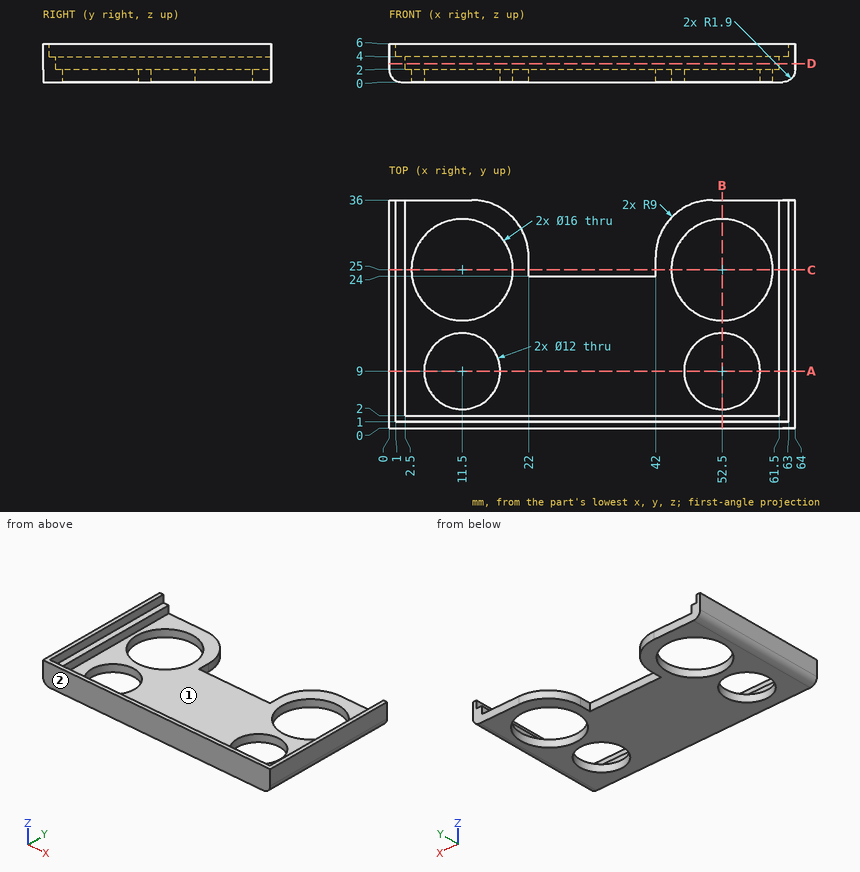
Source: three-view drawing plus pictorial views. Frame: mm from the lowest corner of the part. Round coordinates to 2 decimals unless told otherwise and drop trailing zeros. Order: outer loops, then holes, each group sorted by start corner. A loop starts at its lowest first (then second) coordinate and runs counter-clockwise, first axis right, second up. Notation, with made-up numbers: (-13, 88) - (40, 88) arc R24 cw to (40, 119) - close; hole circle Ø5 at (0, 85.5). An arc over 180 degrees is marked (long way). Use a Markdown table: item, result.
1. Mould query, pull axis X, two halves, no side actions, for the marked faces 1 and 2. Classes: +X half, -X half, draft (parallel to the pull), parting line (faces both ways), or undercut.
Evaluation:
| item | result |
|---|---|
| face 1 | undercut |
| face 2 | draft |
2. First-contact query: pin 1 (1.6 mm diameter, centred on y = 25.5, z = 1, fed in from +X); pin 2 (1.5 mm diameter, centred on x = 27, z = 2, fed in from -Y); pin 3 (18.5 mm diameter, centred on x = 11.5, y = 25, fed in from +Z); pin 4 (17 mm diameter, centred on x = 37, y = 19.5, fed in from +Z). Flat tips, straight axial feed; report the tip coordinate or a pass-through.
Evaluation:
| item | result |
|---|---|
| pin 1 | x = 64 |
| pin 2 | y = 0 |
| pin 3 | z = 4 |
| pin 4 | z = 2 |
3. Section C-C on y = 25. Return the cut outline in (x, z), then the cut area to 3 significant figures.
Evaluation:
| item | result |
|---|---|
| outline | (0, 1.9) arc R1.9 ccw to (1.9, 0) - (3.5, 0) - (3.5, 2) - (2.5, 2) - (2.5, 4) - (1, 4) - (1, 6) - (0, 6) - close; (19.5, 0) - (22, 0) - (22, 2) - (19.5, 2) - close; (42, 0) - (44.5, 0) - (44.5, 2) - (42, 2) - close; (60.5, 0) - (62.1, 0) arc R1.9 ccw to (64, 1.9) - (64, 6) - (63, 6) - (63, 4) - (61.5, 4) - (61.5, 2) - (60.5, 2) - close |
| area | 36.5 mm^2 |
4. Section B-B on x = 52.5. Return the cut outline in (y, z), then the cut area to 3 significant figures.
Evaluation:
| item | result |
|---|---|
| outline | (0, 0) - (3, 0) - (3, 2) - (2, 2) - (2, 4) - (1, 4) - (1, 6) - (0, 6) - close; (15, 0) - (17, 0) - (17, 2) - (15, 2) - close; (33, 0) - (36, 0) - (36, 2) - (33, 2) - close |
| area | 22.0 mm^2 |
5. Material intervals for probe 1 along Y at (x, z) = (52.5, 0.95); probe 2 along X at (y, z) = (6, 1.8); probe 3 along X at (y, z) = (27, 2.8), sorted ascending.
Evaluation:
| item | result |
|---|---|
| probe 1 | 0 to 3, 15 to 17, 33 to 36 |
| probe 2 | 0 to 6.3, 16.7 to 47.3, 57.7 to 64 |
| probe 3 | 0 to 2.5, 61.5 to 64 |
6. Section D-D on z = 2.9. Return the cut outline in (x, y).
Evaluation:
| item | result |
|---|---|
| outline | (0, 0) - (64, 0) - (64, 36) - (61.5, 36) - (61.5, 2) - (2.5, 2) - (2.5, 36) - (0, 36) - close |
7. Section A-A on y = 9. Return the cut outline in (x, z).
Evaluation:
| item | result |
|---|---|
| outline | (0, 1.9) arc R1.9 ccw to (1.9, 0) - (5.5, 0) - (5.5, 2) - (2.5, 2) - (2.5, 4) - (1, 4) - (1, 6) - (0, 6) - close; (17.5, 0) - (46.5, 0) - (46.5, 2) - (17.5, 2) - close; (58.5, 0) - (62.1, 0) arc R1.9 ccw to (64, 1.9) - (64, 6) - (63, 6) - (63, 4) - (61.5, 4) - (61.5, 2) - (58.5, 2) - close |
